```python
from build123d import *

# Parameters (mm, degrees)
F0_W     = 32.8638516366
F0_H     = 19.1183499992
F1_DEPTH = 25
F2_DEPTH = 3
F3_DEPTH = 14


with BuildPart() as f1:
    # F0 (on Top) → F1 (new body)
    with BuildSketch(Plane.XY):
        Polygon((33.5817799435, 0), (33.5817799435, 30), (-33.5817799435, 30), (-33.5817799435, 0), (-16.4319258183, 0), (-16.4319258183, 19.1183499992), (16.4319258183, 19.1183499992), (16.4319258183, 0), align=None)
        with Locations((0, 9.5591749996)):
            Rectangle(F0_W, F0_H)
        with BuildLine():
            Line((16.4319258183, -13.1183499992), (16.4319258183, 0))
            Line((16.4319258183, 0), (-16.4319258183, 0))
            Line((-16.4319258183, 0), (-16.4319258183, -13.1183499992))
            ThreePointArc((-16.4319258183, -13.1183499992), (-12.1892851312, -14.8757093121), (-10.4319258183, -19.1183499992))
            Line((-10.4319258183, -19.1183499992), (10.4319258183, -19.1183499992))
            ThreePointArc((10.4319258183, -19.1183499992), (12.1892851312, -14.8757093121), (16.4319258183, -13.1183499992))
        make_face()
        with BuildLine():
            Line((33.5817799435, -30), (33.5817799435, 0))
            Line((33.5817799435, 0), (16.4319258183, 0))
            Line((16.4319258183, 0), (16.4319258183, -13.1183499992))
            ThreePointArc((16.4319258183, -13.1183499992), (20.6745665054, -14.8757093121), (22.4319258183, -19.1183499992))
            ThreePointArc((22.4319258183, -19.1183499992), (16.4319258183, -25.1183499992), (10.4319258183, -19.1183499992))
            Line((10.4319258183, -19.1183499992), (-10.4319258183, -19.1183499992))
            ThreePointArc((-10.4319258183, -19.1183499992), (-20.6745665054, -23.3609906863), (-16.4319258183, -13.1183499992))
            Line((-16.4319258183, -13.1183499992), (-16.4319258183, 0))
            Line((-16.4319258183, 0), (-33.5817799435, 0))
            Line((-33.5817799435, 0), (-33.5817799435, -30))
            Line((-33.5817799435, -30), (33.5817799435, -30))
        make_face()
    extrude(amount=F1_DEPTH)

    # F0 (on Top) → F2 (join)
    with BuildSketch(Plane.XY):
        with BuildLine():
            Line((-16.4319258183, -15.6183499992), (-16.4319258183, -13.1183499992))
            ThreePointArc((-16.4319258183, -13.1183499992), (-20.6745665054, -23.3609906863), (-10.4319258183, -19.1183499992))
            Line((-10.4319258183, -19.1183499992), (-12.9319258183, -19.1183499992))
            ThreePointArc((-12.9319258183, -19.1183499992), (-18.9067995525, -21.5932237333), (-16.4319258183, -15.6183499992))
        make_face()
        with BuildLine():
            ThreePointArc((-10.4319258183, -19.1183499992), (-12.1892851312, -14.8757093121), (-16.4319258183, -13.1183499992))
            Line((-16.4319258183, -13.1183499992), (-16.4319258183, -15.6183499992))
            ThreePointArc((-16.4319258183, -15.6183499992), (-13.9570520842, -16.643476265), (-12.9319258183, -19.1183499992))
            Line((-12.9319258183, -19.1183499992), (-10.4319258183, -19.1183499992))
        make_face()
        with BuildLine():
            Line((16.4319258183, -15.6183499992), (16.4319258183, -13.1183499992))
            ThreePointArc((16.4319258183, -13.1183499992), (12.1892851312, -14.8757093121), (10.4319258183, -19.1183499992))
            Line((10.4319258183, -19.1183499992), (12.9319258183, -19.1183499992))
            ThreePointArc((12.9319258183, -19.1183499992), (13.9570520842, -16.643476265), (16.4319258183, -15.6183499992))
        make_face()
        with BuildLine():
            ThreePointArc((22.4319258183, -19.1183499992), (20.6745665054, -14.8757093121), (16.4319258183, -13.1183499992))
            Line((16.4319258183, -13.1183499992), (16.4319258183, -15.6183499992))
            ThreePointArc((16.4319258183, -15.6183499992), (18.9067995525, -16.643476265), (19.9319258183, -19.1183499992))
            ThreePointArc((19.9319258183, -19.1183499992), (16.4319258183, -22.6183499992), (12.9319258183, -19.1183499992))
            Line((12.9319258183, -19.1183499992), (10.4319258183, -19.1183499992))
            ThreePointArc((10.4319258183, -19.1183499992), (16.4319258183, -25.1183499992), (22.4319258183, -19.1183499992))
        make_face()
    extrude(amount=F2_DEPTH)

    # F0 (on Top) → F3 (cut)
    with BuildSketch(Plane.XY):
        Polygon((33.5817799435, 0), (33.5817799435, 30), (-33.5817799435, 30), (-33.5817799435, 0), (-16.4319258183, 0), (-16.4319258183, 19.1183499992), (16.4319258183, 19.1183499992), (16.4319258183, 0), align=None)
        with Locations((0, 9.5591749996)):
            Rectangle(F0_W, F0_H)
    extrude(amount=F3_DEPTH, mode=Mode.SUBTRACT)


solid = f1.part
```
Model file for the job. Use its own axes, mm. A direction names the side the tool comes from. Give positions to 0.01 mm unless a question says otherwise; leave off trailing zeros. Order: outer loops, then holes, each group sorted by start corner. A loop starts at its lowest first (then second) coordinate and runs counter-clockwise, first axis right, second up.
1) 3-axis set-ups, long thin cutter, end or side, ignore diameter. For faces 1 (the flat face through (19, -22, 3)), 2 (the flat face through (0, 30, 19)), 3 (the flat face through (0, 0, 7)): which of +Z, -Z, +X, -X, +Y, -Y reach the whole face in a straight line?
2) Wall check: probe 1 along Y at (x, z) = (16.5, 19); probe 2 along X at (y, z) = (-15, 20.75); probe 3 along X at (y, z) = (-18, 23.25). Give the ranges that are in metal, low to high.
3) Saw through at C-C, the plane y = 22.5. Write the cut outline in (x, z).
4) Saw through at A-A, the plane z = 15. Write the cut outline in (x, y).
5) Pin check, flat tips, straight feed: pin 1 (7 mm diameter, centred on x = 4, z = 9.5, fed in from +Y); pin 2 (9 mm diameter, centred on x = 10, y = 11.5, fed in from -Z); pin 3 (2 mm diameter, centred on y = 2, z = 5, fed in from +X). Stop position of each tip, or through.
6) Saw through at D-D, the plane z = 10.25. Write the cut outline in (x, y).
7) Mould opens along Y. For faces 4 (the flat face through (33.582, -7, 15)), 5 (the flat face through (-14, -22, 3)), 6 (the flat face through (0, -30, 12)) say: +Y half, -Y half, draft (parallel to the pull), parting line (faces both ways), or undercut.
8) Saw through at B-B, the plane x = 26.5. Write the cut outline in (y, z), then the cut area to 3 significant figures.
Computed:
1. face 1: +Z
1. face 2: +Z, -Z, +X, -X, +Y
1. face 3: -Z, +X, -X, +Y
2. probe 1: y = -30 to -25.12, -13.12 to 30
2. probe 2: x = -33.58 to -20.8, -12.07 to 12.07, 20.8 to 33.58
2. probe 3: x = -33.58 to -22.33, -10.54 to 10.54, 22.33 to 33.58
3. outline: (-33.58, 14) - (33.58, 14) - (33.58, 25) - (-33.58, 25) - close
4. outline: (-33.58, -30) - (33.58, -30) - (33.58, 30) - (-33.58, 30) - close; hole circle Ø12 at (-16.43, -19.12); hole circle Ø12 at (16.43, -19.12)
5. pin 1: stops at y = 0
5. pin 2: stops at z = 14
5. pin 3: passes through
6. outline: (-33.58, -30) - (33.58, -30) - (33.58, 0) - (-33.58, 0) - close; hole circle Ø12 at (-16.43, -19.12); hole circle Ø12 at (16.43, -19.12)
7. face 4: draft
7. face 5: undercut
7. face 6: -Y half
8. outline: (-30, 0) - (0, 0) - (0, 14) - (30, 14) - (30, 25) - (-30, 25) - close
8. area: 1,080 mm2
